Check sheet for the modelled part. Datum: model origin and axes. Units: mm. A direction names the side the tool comes from. Round coordinates to 2 decimals unless told otherwise and drop trailing zeros. Write each loop counter-clockwise with the first axis right and the second up, starting at its lowest first coordinate (ties: lowest second). Pieces come first, ordered by that corner, then holes. Notation, with made-up numbers: (20, 60) - (76, 60) arc R26 cw to (76, 92) - close; hole circle Ø4 at (37.5, -39.5). An arc over 180 degrees is marked (long way). Use one line per item in the form item = value. Start each with the question number.
1) Scan lines: probe 1 along Z at (x, y) = (15, 2); probe 2 along Y at (x, z) = (75, 6.5); probe 3 along Y at (x, z) = (30, 13.25). Record each from-to range of solid material in increasing order.
2) Section check C-C (y = 44). Record the boundary of the cut face in (x, z), then the cut area to 3 significant figures.
3) Section check A-A (z = 15). Record the boundary of the cut face in (x, y).
4) Section check D-D (z = 23.25). Record the boundary of the cut face in (x, y).
5) Section check B-B (x = 15). Record the boundary of the cut face in (y, z), then the cut area to 3 significant figures.
6) Gauge pin test, flat ends, axial feed: P1, Ø2, axis at x = 125, z = 19, coming from the +Y side; P2, Ø6, axis at x = 55, z = 7.5, coming from the -Y side; P3, Ø1, axis at y = 18, z = 19.5, coming from the -X side; P4, Ø17.5, axis at x = 15, z = 15, coming from the -Y side. Record the tip position at first contact, or that the pin passes through.
7) Draft check along Y on faces 1 (the face through (125, 0, 15)), 2 (the face through (74.276, 46.572, 14.79)), 3 (the face through (150, 2, 15)). Enter one of: +Y half, -Y half, draft (parallel to the pull), parting line (faces both ways), or undercut.
8) Set-up check for faces 4 (the face through (94.671, 3.243, 14.79)), 5 (the face through (128.765, 2.465, 17.585)), 6 (the face through (124, 5, 15)), 7 (the face through (26, 5, 15)), 8 (the face through (25, 0, 15)): record each of +Z, -Z, +X, -X, +Y, -Y from which the full face is reachable in a straight line by a thin tool's end or side.
from build123d import *

# Parameters (mm, degrees)
BOSS_EXTRUDE1_DEPTH   = 30
M12_CLEARANCE_HOLE2_D = 13.5


with BuildPart() as part:
    # Sketch1 → Boss-Extrude1 (new body)
    with BuildSketch(Plane.XY):
        with BuildLine():
            Line((0, 0), (50, 0))
            ThreePointArc((50, 0), (55.286764074, 3.162725669), (55, 9.31662479))
            ThreePointArc((55, 9.31662479), (75, 46.583123952), (95, 9.31662479))
            ThreePointArc((95, 9.31662479), (94.713235926, 3.162725669), (100, 0))
            Line((100, 0), (150, 0))
            Line((150, 0), (150, 5))
            Line((150, 5), (98.061521027, 5))
            ThreePointArc((98.061521027, 5), (75, 51.583123952), (51.938478973, 5))
            Line((51.938478973, 5), (5, 5))
            Line((5, 5), (0, 5))
            Line((0, 5), (0, 0))
        make_face()
    extrude(amount=BOSS_EXTRUDE1_DEPTH)

    # M12 Clearance Hole2 (through all)
    with Locations(Plane(origin=(0, 5, 0), x_dir=(1, 0, 0), z_dir=(0, 1, 0))):
        with Locations((15, -15), (135, -15)):
            Hole(M12_CLEARANCE_HOLE2_D / 2)


solid = part.part
Results are:
q1.probe_1 = 0 to 8.25, 21.75 to 30
q1.probe_2 = 46.58 to 51.58
q1.probe_3 = 0 to 5
q2.outline = (55.45, 0) - (64.17, 0) - (64.17, 30) - (55.45, 30) - close; (85.83, 0) - (94.55, 0) - (94.55, 30) - (85.83, 30) - close
q2.area = 523 mm²
q3.outline = (0, 0) - (8.25, 0) - (8.25, 5) - (0, 5) - close; (21.75, 0) - (50, 0) arc R6 ccw to (55, 9.32) arc R24 cw (long way) to (95, 9.32) arc R6 ccw to (100, 0) - (128.25, 0) - (128.25, 5) - (98.06, 5) arc R29 ccw (long way) to (51.94, 5) - (21.75, 5) - close; (141.75, 0) - (150, 0) - (150, 5) - (141.75, 5) - close
q4.outline = (0, 0) - (50, 0) arc R6 ccw to (55, 9.32) arc R24 cw (long way) to (95, 9.32) arc R6 ccw to (100, 0) - (150, 0) - (150, 5) - (98.06, 5) arc R29 ccw (long way) to (51.94, 5) - (0, 5) - close
q5.outline = (0, 0) - (5, 0) - (5, 8.25) - (0, 8.25) - close; (0, 21.75) - (5, 21.75) - (5, 30) - (0, 30) - close
q5.area = 82.5 mm²
q6.P1 = 5
q6.P2 = 0.34
q6.P3 = 46.29
q6.P4 = 0
q7.face_1 = -Y half
q7.face_2 = undercut
q7.face_3 = draft
q8.face_4 = +Z, -Z
q8.face_5 = +Y, -Y
q8.face_6 = +Z, -Z, +X
q8.face_7 = +Z, -Z, -X
q8.face_8 = +Z, -Z, +X, -X, -Y
